The model under review builds one solid part; all positions refer to its coordinate system, in mm. A direction names the side the tool comes from. Round coordinates to 2 decimals unless told otherwise and drop trailing zeros. Order: outer loops, then holes, each group sorted by start corner. A loop starts at its lowest first (then second) coordinate and runs counter-clockwise, first axis right, second up.
1) Machinability: for faces 4 (the face through (45.91, 1, -2)), 5 (the face through (12.09, 1, -16)), 6 (the face through (23.8, 1, -6)), 7 (the face through (34, 2, -7)), which of the approach directions +Z, -Z, +X, -X, +Y, -Y give a long, thin tool a straight path to every point of the face, cutting with its end or side? Answer none if there is none.
2) To check wall thickness, follow L1, parallel to X at y = 0.5, z = -2; L2, parallel to X at y = 0.4, z = -16; L3, parallel to X at y = 0.3, z = -17. State the ranges of each line that lie inside material, in increasing order.
3) Consider section A-A (z = 2.5). Give the boundary of the cut face in (x, y).
4) Mouldability with a two-part tool opening along Z and no side actions: class faces 1 (the face through (31.3, 1.01, -6.11)), 2 (the face through (22, 1, 5)), 3 (the face through (42.91, 1, -4)) as pulls with the +Z half, pulls with the -Z half, needs draft (parallel to the pull), parting line crosses it, or undercut.
5) Consider section C-C (z = -3). Give the boundary of the cut face in (x, y), then the cut area to 3 significant figures.
6) Consider section B-B (x = 32). Give the boundary of the cut face in (y, z).
7) Clearance check with a flat-ended pin moving along its axis: P1, Ø12, axis at x = 33.5, z = -1, coming from the -Y side. State where the tip first meets the part, or that it passes through.
8) Consider section D-D (z = -9). Give the boundary of the cut face in (x, y).
from build123d import *

# Parameters (mm, degrees)
BOSS_EXTRUDE1_DEPTH = 2
CUT_EXTRUDE1_DEPTH  = 3
FILLET1_R           = 0.2


with BuildPart() as part:
    # Sketch2 → Boss-Extrude1 (new body)
    with BuildSketch(Plane(origin=(0, 0, 0), x_dir=(1, 0, 0), z_dir=(0, 1, 0))):
        with BuildLine():
            Line((0, 0.500000092), (0, 20.455103274))
            ThreePointArc((0, 20.455103274), (4.54489668, 25.000000092), (9.089793452, 20.455103365))
            Line((9.089793452, 20.455103365), (9.089793452, 15.776597525))
            Line((9.089793452, 15.776597525), (4.544896726, 15.776597525))
            Line((4.544896726, 15.776597525), (4.544896726, 11.719673062))
            ThreePointArc((4.544896726, 11.719673062), (8.317345089, 7.947224699), (12.089793452, 11.719673062))
            Line((12.089793452, 11.719673062), (12.089793452, 19.500000092))
            ThreePointArc((12.089793452, 19.500000092), (13.700706156, 23.389087388), (17.589793452, 25.000000092))
            Line((17.589793452, 25.000000092), (27.5, 25.000000092))
            Line((27.5, 25.000000092), (49.5, 25.000000092))
            ThreePointArc((49.5, 25.000000092), (53.389087297, 23.389087388), (55, 19.500000092))
            Line((55, 19.500000092), (55, -0.455103091))
            ThreePointArc((55, -0.455103091), (50.45510332, -4.999999908), (45.910206548, -0.455103182))
            Line((45.910206548, -0.455103182), (45.910206548, 4.223402658))
            Line((45.910206548, 4.223402658), (50.455103274, 4.223402658))
            Line((50.455103274, 4.223402658), (50.455103274, 8.280327121))
            ThreePointArc((50.455103274, 8.280327121), (46.682654911, 12.052775484), (42.910206548, 8.280327121))
            Line((42.910206548, 8.280327121), (42.910206548, 0.500000092))
            ThreePointArc((42.910206548, 0.500000092), (41.299293844, -3.389087205), (37.410206548, -4.999999908))
            Line((37.410206548, -4.999999908), (27.5, -4.999999908))
            Line((27.5, -4.999999908), (5.5, -4.999999908))
            ThreePointArc((5.5, -4.999999908), (1.610912703, -3.389087205), (0, 0.500000092))
        make_face()
    extrude(amount=BOSS_EXTRUDE1_DEPTH)

    # Sketch3 → Cut-Extrude1 (cut, through all)
    with BuildSketch(Plane(origin=(0, 2, 0), x_dir=(1, 0, 0), z_dir=(0, 1, 0))):
        with BuildLine():
            Line((27.5, 2.107265014), (20.001901677, 10.000000092))
            ThreePointArc((20.001901677, 10.000000092), (20.810460493, 16.947460398), (27.5, 14.905149634))
            ThreePointArc((27.5, 14.905149634), (34.189539507, 16.947460398), (34.998098323, 10.000000092))
            Line((34.998098323, 10.000000092), (27.5, 2.107265014))
        make_face()
    extrude(amount=-CUT_EXTRUDE1_DEPTH, mode=Mode.SUBTRACT)

    # Fillet1
    fillet1_edges = [part.edges().sort_by_distance(p)[0] for p in [
        (27.5, 1, -14.905149634),
    ]]
    fillet(fillet1_edges, radius=FILLET1_R)


solid = part.part
Answer below:
1. face 4: +Z, +Y, -Y
1. face 5: -Z, +Y, -Y
1. face 6: +Y, -Y
1. face 7: +Z, -Z, +X, -X, +Y
2. L1: x = 0 to 42.91, 45.91 to 55
2. L2: x = 0 to 9.09, 12.09 to 19.76, 26.84 to 28.16, 35.24 to 55
2. L3: x = 0 to 9.09, 12.09 to 20.89, 25.71 to 29.29, 34.11 to 55
3. outline: (0.89, 0) - (42.02, 0) - (42.02, 2) - (0.89, 2) - close; (46.4, 0) - (54.51, 0) - (54.51, 2) - (46.4, 2) - close
4. face 1: undercut
4. face 2: pulls with the +Z half
4. face 3: needs draft
5. outline: (0, 0) - (26.65, 0) - (26.65, 2) - (0, 2) - close; (28.35, 0) - (42.91, 0) - (42.91, 2) - (28.35, 2) - close; (45.91, 0) - (55, 0) - (55, 2) - (45.91, 2) - close
5. area: 101 mm2
6. outline: (0, -25) - (2, -25) - (2, -17.68) - (0, -17.68) - close; (0, -6.84) - (2, -6.84) - (2, 5) - (0, 5) - close
7. P1: stops at y = 0
8. outline: (0, 0) - (5.7, 0) - (5.7, 2) - (0, 2) - close; (10.93, 0) - (20.95, 0) - (20.95, 2) - (10.93, 2) - close; (34.05, 0) - (42.98, 0) - (42.98, 2) - (34.05, 2) - close; (50.39, 0) - (55, 0) - (55, 2) - (50.39, 2) - close
